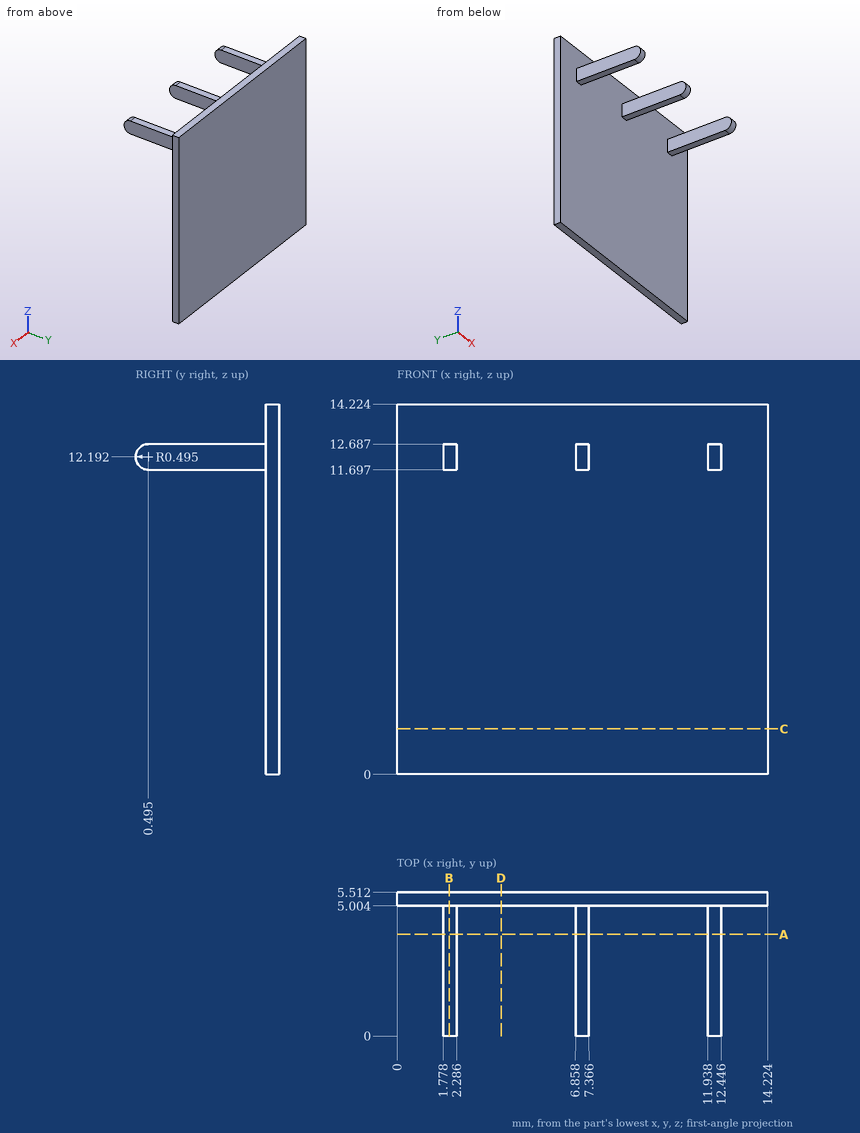
Print and shaded views of the part. All mm, measured from the part's lowest x, y and z. Coordinates: 2 decimals unless noted, no trailing zeros. Order: outer loops, then holes, each group sorted by start corner. A loop starts at its lowest first (then second) coordinate and runs counter-clockwise, first axis right, second up. Notation, with made-up numbers: M -28.5,52 L 22.5,52 A37 ccw 22.5,91 Z; hole C -21,86.5 d8. An arc over 180 degrees is marked long. Write each question's results on one line, items separated by ' | '. Start each with the question number.
Q1. Cut at C-C (z = 1.75). List the corners of the cut face in (x, y).
Q2. Cut at D-D (x = 4). List the corners of the cut face in (y, z).
Q3. Flat gauge pins, fed straight in: P1, Ø0.6, axis at x = 7, y = 3, coming from the -Z side; P2, Ø1.1, axis at y = 2, z = 12, coming from the -X side; P3, Ø1.1, axis at y = 3.5, z = 12, coming from the +X side. Where does each tip first touch, or does it go through?
Q4. Cut at B-B (x = 2). List the corners of the cut face in (y, z) (1 decimal), then the cut area to 3 significant figures.
Q5. Cut at A-A (y = 3.9). List the corners of the cut face in (x, z).
Q6. Drill centre lines: probe 1 along Y at (x, z) = (4, 13.75); probe 2 along Z at (x, y) = (7, 4.4). Where is each one in solid material? Low to high. Write a range as from..to.
Found:
1) outline: M 0,5 L 14.22,5 L 14.22,5.51 L 0,5.51 Z
2) outline: M 5,0 L 5.51,0 L 5.51,14.22 L 5,14.22 Z
3) P1: z = 11.7 | P2: x = 1.78 | P3: x = 12.45
4) outline: M 0.5,11.7 L 5,11.7 L 5,0 L 5.5,0 L 5.5,14.2 L 5,14.2 L 5,12.7 L 0.5,12.7 A0.5 ccw Z | area: 12.1 mm²
5) outline: M 1.78,11.7 L 2.29,11.7 L 2.29,12.69 L 1.78,12.69 Z; M 6.86,11.7 L 7.37,11.7 L 7.37,12.69 L 6.86,12.69 Z; M 11.94,11.7 L 12.45,11.7 L 12.45,12.69 L 11.94,12.69 Z
6) probe 1: 5..5.51 | probe 2: 11.7..12.69
